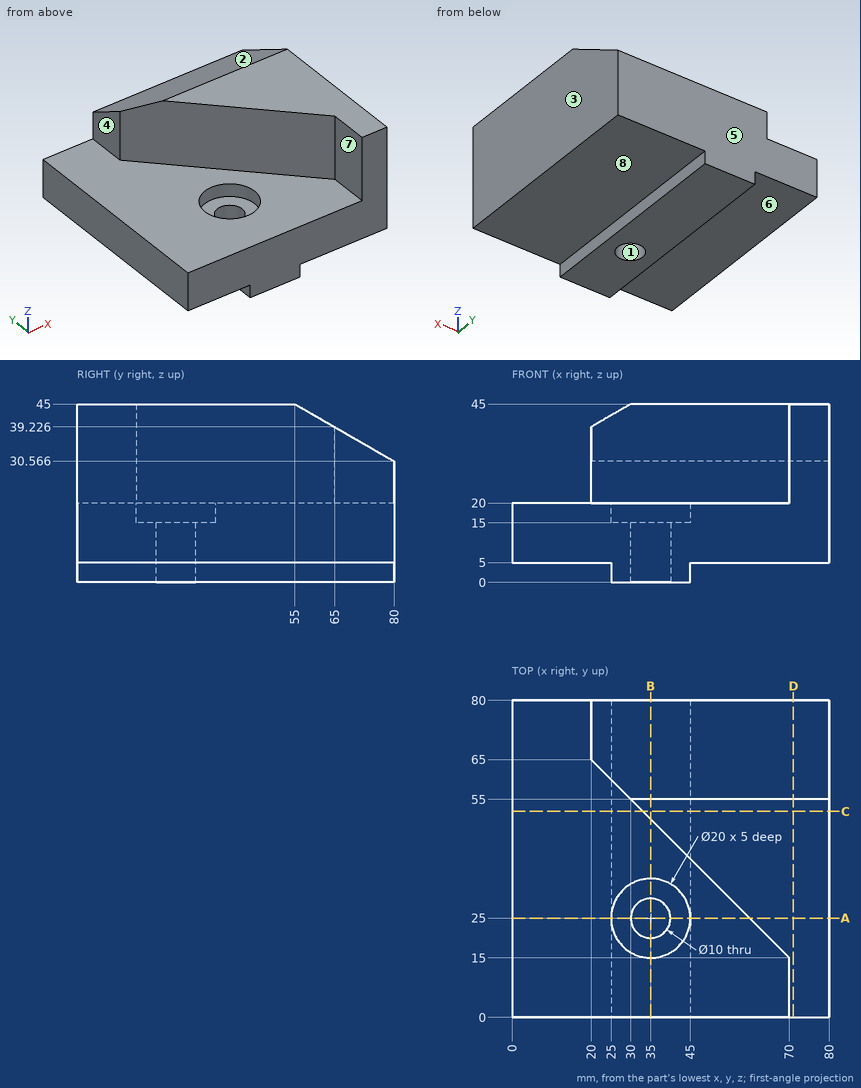
Geometry: see drawing. Coordinates: mm, zero at the bounding-box minimum. A direction names the side the tool comes from. Coordinates: 2 decimals unless noted, no trailing zeros. Loops run counter-clockwise (first coordinate to the right, second up) from the corner with the lowest first, then second, coordinate; pieces in that order, holes last.
(1) Section B-B on x = 35. Return the cut outline in (y, z), then the cut area to 3 significant figures.
(2) Section D-D on x = 71. Return the cut outline in (y, z), then the cut area to 3 significant figures.
(3) Section C-C on y = 52. Return the cut outline in (x, z).
(4) Section A-A on y = 25. Return the cut outline in (x, z).
(5) Set-up query: the marked faces 5, 6, 7 and 8. Return all of +Z, -Z, +X, -X, +Y, -Y with unobstructed straight access to the full face (end or side cutting, diameter ignored); none if empty.
(6) Material intervals for probe 1 along Y at (x, z) = (35, 10); probe 2 along X at (y, z) = (67, 4); probe 3 along Z at (x, y) = (9, 40.5), sorted ascending.
(7) First-contact query: pin 1 Ø16.5 at (y, z) = (71.5, 29.5) entering from -X; pin 2 Ø10 at (x, y) = (32, 20.5) entering from +Z; pin 3 Ø1.5 at (y, z) = (43.5, 2.5) entering from -X. Flat tips, straight axial feed; report the tip coordinate or a pass-through.
(8) Pull-direction query (X, two-part tool) for the marked faces 1, 2, 3 and 4; classes: released by +X, released by -X, zero draft, split by the parting line, or undercut.
Data:
1. outline: (0, 0) - (20, 0) - (20, 15) - (15, 15) - (15, 20) - (0, 20) - close; (30, 0) - (80, 0) - (80, 30.57) - (55, 45) - (50, 45) - (50, 20) - (35, 20) - (35, 15) - (30, 15) - close
1. area: 1,920 mm2
2. outline: (0, 5) - (80, 5) - (80, 30.57) - (55, 45) - (0, 45) - close
2. area: 3,020 mm2
3. outline: (0, 5) - (25, 5) - (25, 0) - (45, 0) - (45, 5) - (80, 5) - (80, 45) - (33, 45) - (33, 20) - (0, 20) - close
4. outline: (0, 5) - (25, 5) - (25, 0) - (30, 0) - (30, 15) - (25, 15) - (25, 20) - (0, 20) - close; (40, 0) - (45, 0) - (45, 5) - (80, 5) - (80, 45) - (60, 45) - (60, 20) - (45, 20) - (45, 15) - (40, 15) - close
5. face 5: +Z, -Z, +X, -X, +Y
5. face 6: -Z, -X, +Y, -Y
5. face 7: +Z, -X, -Y
5. face 8: -Z, +X, +Y, -Y
6. probe 1: y = 0 to 20, 30 to 80
6. probe 2: x = 25 to 45
6. probe 3: z = 5 to 20
7. pin 1: stops at x = 20
7. pin 2: stops at z = 20
7. pin 3: stops at x = 25
8. face 1: undercut
8. face 2: zero draft
8. face 3: released by +X
8. face 4: released by -X
